Job drawing, mm, ordinate dimensions from the low corner. One solid piece. Give positions to 0.01 mm unless a question says otherwise; leave off trailing zeros. Order: outer loops, then holes, each group sorted by start corner. A loop starts at its lowest first (then second) coordinate and runs counter-clockwise, first axis right, second up. Notation, with made-up numbers: M -8,37.25 L 50,37.25 A17 cw 50,42.25 Z; hole C 15.25,40.25 d9. An arc over 180 degrees is marked long. Put each result on its own line as item: value. Start each with the question number.
1) Pin check, flat tips, straight feed: pin 1 (8 mm diameter, centred on x = 57, y = 31, fed in from -Z); pin 2 (4 mm diameter, centred on x = 34.5, z = 74, fed in from -Y); pin 3 (5 mm diameter, centred on x = 29.5, z = 43.5, fed in from -Y); pin 4 (2 mm diameter, centred on x = 50.5, y = 13, fed in from -Z). Stop position of each tip, or through.
2) Cut at A-A (x = 35). Write the cut outline in (y, z), and give its area (3 significant figures).
3) Cut at D-D (x = 50.5). Write the cut outline in (y, z).
4) Two-plate mould, pull along X, no slides. Class the marked faces 1, 2, 3 and 4: released by +X, released by -X, zero draft, split by the parting line, or undercut.
5) Cut at C-C (z = 12.5). Write the cut outline in (x, y), and give its area (3 significant figures).
6) Drill centre lines: line 1 (Y direction, x = 35, z = 17); line 2 (Y direction, x = 35, z = 93.5); line 3 (Z direction, x = 11, y = 18). Where is each one in solid material? Low to high. Write a range as [from, to].
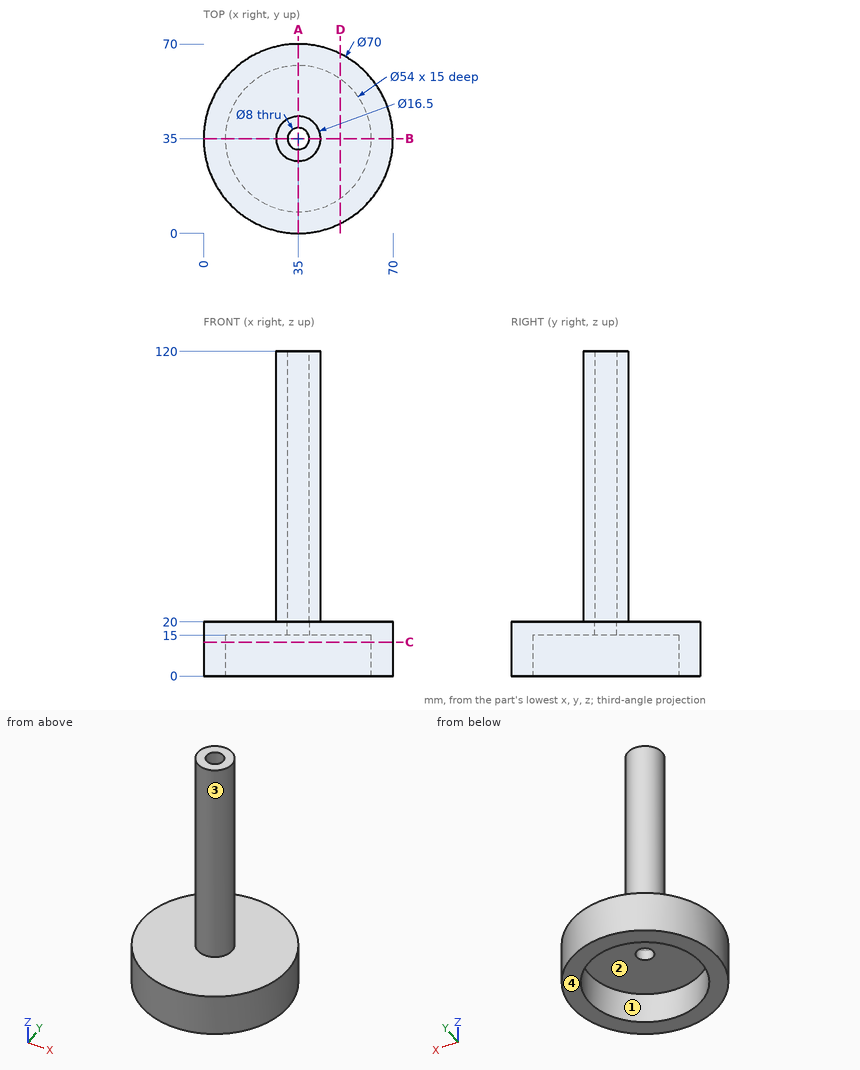
Solution:
1. pin 1: z = 15
1. pin 2: y = 26.75
1. pin 3: y = 27.31
1. pin 4: z = 0
2. outline: M 0,0 L 8,0 L 8,15 L 31,15 L 31,120 L 26.75,120 L 26.75,20 L 0,20 Z; M 39,15 L 62,15 L 62,0 L 70,0 L 70,20 L 43.25,20 L 43.25,120 L 39,120 Z
2. area: 1,400 mm²
3. outline: M 3.62,0 L 12.89,0 L 12.89,15 L 57.11,15 L 57.11,0 L 66.38,0 L 66.38,20 L 3.62,20 Z
4. face 1: undercut
4. face 2: undercut
4. face 3: split by the parting line
4. face 4: zero draft
5. outline: C 35,35 d70; hole C 35,35 d54
5. area: 1,560 mm²
6. line 1: [0, 31], [39, 70]
6. line 2: [26.75, 31], [39, 43.25]
6. line 3: [0, 20]
